Build history of the part. All positions in model axes, mm. Face numbers are marked on the shaded views. A direction names the side the tool comes from. Round coordinates to 2 decimals unless told otherwise and drop trailing zeros. Loops run counter-clockwise (first coordinate to the right, second up) from the corner with the lowest first, then second, coordinate; pieces in that order, holes last. Notation, with made-up numbers: (13.25, -37) - (43.25, -37) arc R22 ccw to (43.25, -20) - close; hole circle Ø3 at (-9.75, 81). An arc over 180 degrees is marked (long way). Use a Markdown table: item, result.
from build123d import *
from OCP.BRepFilletAPI import BRepFilletAPI_MakeChamfer

# Parameters (mm, degrees)
SKETCH1_R                    = 20
BOSS_EXTRUDE1_DEPTH          = 40
WRAP6_SECTION_W              = 2
WRAP6_SECTION_H              = 40
WRAP6_ANGLE                  = 68.754935416
CUT_EXTRUDE3_DEPTH           = 40
CUT_EXTRUDE4_DEPTH           = 40
SHELL1_START                 = -38.5
SHELL1_DEPTH                 = 37
BOSS_EXTRUDE6_DEPTH          = 1.7
CHAMFER3_SIZE2               = 5.104153638
CHAMFER3_SIZE                = 0.9
LPATTERN3_COUNT              = 7
LPATTERN3_PITCH              = 6.22
CHAMFER3_OF_LPATTERN3_SIZE   = 0.9
CHAMFER3_OF_LPATTERN3_SIZE_2 = 5.104153638
BOSS_EXTRUDE9_DEPTH          = 1.7
BOSS_EXTRUDE10_DEPTH         = 1.7
BOSS_EXTRUDE11_REACH         = 61.927
BOSS_EXTRUDE11_END_RADIUS    = 20
SKETCH26_W                   = 1.7
SKETCH26_H                   = 8.060132267
BOSS_EXTRUDE12_REACH         = 61.482
BOSS_EXTRUDE12_END_RADIUS    = 20
SKETCH31_W                   = 1.7
SKETCH31_H                   = 8.563925154
SKETCH35_R                   = 2.4
CUT_EXTRUDE5_DEPTH           = 46.6949855
SKETCH36_R                   = 3.1
CUT_EXTRUDE6_DEPTH           = 0.4
CUT_EXTRUDE7_START           = -0.4
SKETCH37_R                   = 3.1
CUT_EXTRUDE7_DEPTH           = 0.4
LPATTERN4_COUNT              = 2
LPATTERN4_PITCH              = 16
FILLET1_R                    = 4
BOSS_EXTRUDE13_DEPTH         = 0.4
LPATTERN5_COUNT              = 2
LPATTERN5_PITCH              = 40.1
SKETCH39_W                   = 40.5
SKETCH39_H                   = 1.5
BOSS_EXTRUDE14_DEPTH         = 1.5
SKETCH40_W                   = 40.5
SKETCH40_H                   = 1.5
BOSS_EXTRUDE15_DEPTH         = 2
BOSS_EXTRUDE15_TAPER         = 12


# Read off the part's stored shape, not the designer's step: Shell1
with BuildPart() as part:
    # Sketch1 → Boss-Extrude1 (new body)
    with BuildSketch(Plane(origin=(0, 0, 0), x_dir=(0, 0, -1), z_dir=(1, 0, 0))):
        Circle(SKETCH1_R)
    extrude(amount=-BOSS_EXTRUDE1_DEPTH)

    # Wrap6 section (on wrap section) → Wrap6 (revolve)
    with BuildSketch(Plane(origin=(0, 0, 0), x_dir=(0, 0.19866933079506122, 0.9800665778412416), z_dir=(0, 0.9800665778412416, -0.19866933079506122))):
        with Locations((21, -20)):
            Rectangle(WRAP6_SECTION_W, WRAP6_SECTION_H)
    revolve(axis=Axis((0, 0, 0), (1, 0, 0)), revolution_arc=WRAP6_ANGLE)

    # Sketch7 → Cut-Extrude3 (cut)
    with BuildSketch(Plane(origin=(0, 0, 0), x_dir=(0, 0, -1), z_dir=(1, 0, 0))):
        Polygon((-21.561464713, 4.370725277), (-10.806046117, -16.829419696), (-13.2224557, -32.299256077), (-33.361013034, 4.370725277), align=None)
    extrude(amount=-CUT_EXTRUDE3_DEPTH, mode=Mode.SUBTRACT)

    # Sketch8 → Cut-Extrude4 (cut)
    with BuildSketch(Plane(origin=(0, 0, 0), x_dir=(0, 0, -1), z_dir=(1, 0, 0))):
        with BuildLine():
            Line((-19.601331557, 3.973386616), (-17.669228411, 0))
            Line((-17.669228411, 0), (20, 0))
            ThreePointArc((20, 0), (1.996668333, 19.900083306), (-19.601331557, 3.973386616))
        make_face()
    extrude(amount=-CUT_EXTRUDE4_DEPTH, mode=Mode.SUBTRACT)

    # Shell1 outline → Shell1 (cut)
    with BuildSketch(Plane.YZ.offset(SHELL1_START)):
        with BuildLine():
            Line((0, 17.662079948), (-15.779750214, 9.656577198))
            ThreePointArc((-15.779750214, 9.656577198), (-16.138411913, -9.044427064), (0, -18.5))
            Line((0, -18.5), (0, 17.662079948))
        make_face()
    extrude(amount=SHELL1_DEPTH, mode=Mode.SUBTRACT)

    # Sketch17 → Boss-Extrude6 (add)
    with BuildSketch(Plane(origin=(0, -7.804938117, 15.384414667), x_dir=(1, 0, 0), z_dir=(0, -0.4524337453692514, 0.8917980186405168))):
        Polygon((-2.641259026, 11.553646958), (0, 11.553646958), (0, 13.652938378), (0, 17.652938378), (-2.641259026, 17.652938378), align=None)
    boss_extrude6 = extrude(amount=-BOSS_EXTRUDE6_DEPTH)

    # Chamfer3
    chamfer3_edges = [part.edges().sort_by_distance(p)[0] for p in [
        (-1.320629513, 8.707054719, 21.855143062),
    ]]
    chamfer3_side = [part.faces().sort_by_distance(p)[0] for p in [
        (-1.320629513, 8.698910912, 21.871195427),
    ]]
    chamfer(chamfer3_edges, length=CHAMFER3_SIZE - 0.0001, length2=CHAMFER3_SIZE2 - 0.0001, reference=chamfer3_side[0])  # a hair under: the kernel refuses the full size

    # LPattern3: Boss-Extrude6 ×7
    with Locations(*[(-i * LPATTERN3_PITCH, 0, 0) for i in range(1, LPATTERN3_COUNT)]):
        add(boss_extrude6)

    # Chamfer3 of LPattern3
    chamfer3_of_lpattern3_edges_1 = [part.edges().sort_by_distance(p)[0] for p in [
        (-7.540629513, 8.707054719, 21.855143062),
    ]]
    chamfer3_of_lpattern3_side_1 = [part.faces().sort_by_distance(p)[0] for p in [
        (-7.540629513, 8.698910912, 21.871195427),
    ]]
    chamfer3_of_lpattern3_edges_2 = [part.edges().sort_by_distance(p)[0] for p in [
        (-13.760629513, 8.707054719, 21.855143062),
    ]]
    chamfer3_of_lpattern3_side_2 = [part.faces().sort_by_distance(p)[0] for p in [
        (-13.760629513, 8.698910912, 21.871195427),
    ]]
    chamfer3_of_lpattern3_edges_3 = [part.edges().sort_by_distance(p)[0] for p in [
        (-19.980629513, 8.707054719, 21.855143062),
    ]]
    chamfer3_of_lpattern3_side_3 = [part.faces().sort_by_distance(p)[0] for p in [
        (-19.980629513, 8.698910912, 21.871195427),
    ]]
    chamfer3_of_lpattern3_edges_4 = [part.edges().sort_by_distance(p)[0] for p in [
        (-26.200629513, 8.707054719, 21.855143062),
    ]]
    chamfer3_of_lpattern3_side_4 = [part.faces().sort_by_distance(p)[0] for p in [
        (-26.200629513, 8.698910912, 21.871195427),
    ]]
    chamfer3_of_lpattern3_edges_5 = [part.edges().sort_by_distance(p)[0] for p in [
        (-32.420629513, 8.707054719, 21.855143062),
    ]]
    chamfer3_of_lpattern3_side_5 = [part.faces().sort_by_distance(p)[0] for p in [
        (-32.420629513, 8.698910912, 21.871195427),
    ]]
    chamfer3_of_lpattern3_edges_6 = [part.edges().sort_by_distance(p)[0] for p in [
        (-38.640629513, 8.707054719, 21.855143062),
    ]]
    chamfer3_of_lpattern3_side_6 = [part.faces().sort_by_distance(p)[0] for p in [
        (-38.640629513, 8.691002355, 21.846999255),
    ]]
    chamfer3_of_lpattern3 = BRepFilletAPI_MakeChamfer(part.part.solid().wrapped)
    for e in chamfer3_of_lpattern3_edges_1:
        chamfer3_of_lpattern3.Add(CHAMFER3_OF_LPATTERN3_SIZE - 0.0001, CHAMFER3_OF_LPATTERN3_SIZE_2 - 0.0001, e.wrapped, chamfer3_of_lpattern3_side_1[0].wrapped)
    for e in chamfer3_of_lpattern3_edges_2:
        chamfer3_of_lpattern3.Add(CHAMFER3_OF_LPATTERN3_SIZE - 0.0001, CHAMFER3_OF_LPATTERN3_SIZE_2 - 0.0001, e.wrapped, chamfer3_of_lpattern3_side_2[0].wrapped)
    for e in chamfer3_of_lpattern3_edges_3:
        chamfer3_of_lpattern3.Add(CHAMFER3_OF_LPATTERN3_SIZE - 0.0001, CHAMFER3_OF_LPATTERN3_SIZE_2 - 0.0001, e.wrapped, chamfer3_of_lpattern3_side_3[0].wrapped)
    for e in chamfer3_of_lpattern3_edges_4:
        chamfer3_of_lpattern3.Add(CHAMFER3_OF_LPATTERN3_SIZE - 0.0001, CHAMFER3_OF_LPATTERN3_SIZE_2 - 0.0001, e.wrapped, chamfer3_of_lpattern3_side_4[0].wrapped)
    for e in chamfer3_of_lpattern3_edges_5:
        chamfer3_of_lpattern3.Add(CHAMFER3_OF_LPATTERN3_SIZE - 0.0001, CHAMFER3_OF_LPATTERN3_SIZE_2 - 0.0001, e.wrapped, chamfer3_of_lpattern3_side_5[0].wrapped)
    for e in chamfer3_of_lpattern3_edges_6:
        chamfer3_of_lpattern3.Add(CHAMFER3_OF_LPATTERN3_SIZE_2 - 0.0001, CHAMFER3_OF_LPATTERN3_SIZE - 0.0001, e.wrapped, chamfer3_of_lpattern3_side_6[0].wrapped)
    add(Compound.cast(chamfer3_of_lpattern3.Shape()), mode=Mode.REPLACE)  # a hair under: the kernel refuses the full size



with BuildPart() as body_2:
    # Sketch18 → Boss-Extrude9 (new body)
    with BuildSketch(Plane(origin=(-12, 9.40212228, -3.028508389), x_dir=(0, -0.20791169081773309, -0.9781476007338114), z_dir=(1, 0, 0))):
        with BuildLine():
            Line((24.462887784, -6.44514078), (19.462887784, -6.44514078))
            Line((19.462887784, -6.44514078), (18.368989474, -14.430697657))
            Line((18.368989474, -14.430697657), (24.462887784, -13.44514078))
            ThreePointArc((24.462887784, -13.44514078), (27.962887784, -9.94514078), (24.462887784, -6.44514078))
        make_face()
    boss_extrude9 = extrude(amount=BOSS_EXTRUDE9_DEPTH)


with BuildPart() as body_3:
    # Sketch23 → Boss-Extrude10 (new body)
    with BuildSketch(Plane(origin=(-12, 6.645607303, -3.623209558), x_dir=(0, -0.3420201433256566, -0.9396926207859128), z_dir=(1, 0, 0))):
        with BuildLine():
            Line((23.775411733, -9.543929755), (18.775411733, -9.543929755))
            Line((18.775411733, -9.543929755), (16.378556498, -17.765602275))
            Line((16.378556498, -17.765602275), (23.775411733, -16.543929755))
            ThreePointArc((23.775411733, -16.543929755), (27.275411733, -13.043929755), (23.775411733, -9.543929755))
        make_face()
    boss_extrude10 = extrude(amount=BOSS_EXTRUDE10_DEPTH)


with BuildPart() as part_1:
    add(part.part)

    add(body_2.part)  # Boss-Extrude11 merges body 2
    # Boss-Extrude11: up to this cylinder (the profile starts outside it)
    boss_extrude11_end = Plane(origin=(-11.15, 0, 0), z_dir=(1, 0, 0)) * Cylinder(BOSS_EXTRUDE11_END_RADIUS, 164.854, mode=Mode.PRIVATE)
    # Sketch26 → Boss-Extrude11 (add, up to the surface)
    with BuildSketch(Plane(origin=(0, -6.71453374, -18.65024081), x_dir=(1, 0, 0), z_dir=(0, 0.3387394336586716, 0.9408802240905069)), mode=Mode.PRIVATE) as boss_extrude11_sk1:
        with Locations((-11.15, 2.098020073)):
            Rectangle(SKETCH26_W, SKETCH26_H)
    boss_extrude11_tool1 = extrude(boss_extrude11_sk1.sketch, amount=BOSS_EXTRUDE11_REACH, mode=Mode.PRIVATE) - boss_extrude11_end
    boss_extrude11 = boss_extrude11_tool1.solids().sort_by_distance((-11.15, -4.740548, -19.360923))[0]
    add(boss_extrude11)


    add(body_3.part)  # Boss-Extrude12 merges body 3
    # Boss-Extrude12: up to this cylinder (the profile starts outside it)
    boss_extrude12_end = Plane(origin=(-11.15, 0, 0), z_dir=(1, 0, 0)) * Cylinder(BOSS_EXTRUDE12_END_RADIUS, 163.964, mode=Mode.PRIVATE)
    # Sketch31 → Boss-Extrude12 (add, up to the surface)
    with BuildSketch(Plane(origin=(0, -11.64258856, -15.876784348), x_dir=(-1, 0, 0), z_dir=(0, -0.5913508934195582, -0.8064143605193862)), mode=Mode.PRIVATE) as boss_extrude12_sk1:
        with Locations((11.15, -0.687946115)):
            Rectangle(SKETCH31_W, SKETCH31_H)
    boss_extrude12_tool1 = extrude(boss_extrude12_sk1.sketch, amount=-BOSS_EXTRUDE12_REACH, mode=Mode.PRIVATE) - boss_extrude12_end
    boss_extrude12 = boss_extrude12_tool1.solids().sort_by_distance((-11.15, -12.197358, -15.469967))[0] + boss_extrude12_tool1.solids().sort_by_distance((-11.15, -12.197358, -15.469967))[1]
    add(boss_extrude12)

    # Sketch35 → Cut-Extrude5 (cut, through all)
    with BuildSketch(Plane(origin=(-10.3, 0, 0), x_dir=(0, 0, -1), z_dir=(1, 0, 0))):
        with Locations((24.889112346, -5.411813674)):
            Circle(SKETCH35_R)
        with Locations((21.503501796, -13.743346963)):
            Circle(SKETCH35_R)
    cut_extrude5 = extrude(amount=-CUT_EXTRUDE5_DEPTH, mode=Mode.SUBTRACT)

    # Sketch36 → Cut-Extrude6 (cut)
    with BuildSketch(Plane(origin=(-10.3, 0, 0), x_dir=(0, 0, -1), z_dir=(1, 0, 0))):
        with Locations((24.889112346, -5.411813674)):
            Circle(SKETCH36_R)
        with Locations((21.503501796, -13.743346963)):
            Circle(SKETCH36_R)
    cut_extrude6 = extrude(amount=-CUT_EXTRUDE6_DEPTH, mode=Mode.SUBTRACT)

    # Sketch37 → Cut-Extrude7 (cut)
    with BuildSketch(Plane.ZY.offset(12).offset(CUT_EXTRUDE7_START)):
        with Locations(Location((-24.889112346, -5.411813674, 0), (0, 0, 180))):
            Circle(SKETCH37_R)
        with Locations(Location((-21.503501796, -13.743346963, 0), (0, 0, 180))):
            Circle(SKETCH37_R)
    cut_extrude7 = extrude(amount=CUT_EXTRUDE7_DEPTH, mode=Mode.SUBTRACT)

    # LPattern4: Boss-Extrude9, Boss-Extrude10, Boss-Extrude11, Boss-Extrude12, Cut-Extrude5, Cut-Extrude6, Cut-Extrude7 ×2
    with Locations(*[(-i * LPATTERN4_PITCH, 0, 0) for i in range(1, LPATTERN4_COUNT)]):
        add(boss_extrude9)
        add(boss_extrude10)
        add(boss_extrude11)
        add(boss_extrude12)
        add(cut_extrude5, mode=Mode.SUBTRACT)
        add(cut_extrude6, mode=Mode.SUBTRACT)
        add(cut_extrude7, mode=Mode.SUBTRACT)

    # Fillet1
    fillet1_edges = [part_1.edges().sort_by_distance(p)[0] for p in [
        (-20, -16.829419696, 10.806046117),
    ]]
    fillet(fillet1_edges, radius=FILLET1_R)

    # Sketch38 → Boss-Extrude13 (add)
    with BuildSketch(Plane(origin=(0, 0, 0), x_dir=(0, 0, -1), z_dir=(1, 0, 0))):
        Polygon((-19.72457086, 0.75), (20, 0.75), (20, -0.75), (-16.900694448, -0.75), (-16.986407143, -4.647229987), align=None)
    boss_extrude13 = extrude(amount=BOSS_EXTRUDE13_DEPTH)

    # LPattern5: Boss-Extrude13 ×2
    with Locations(*[(-i * LPATTERN5_PITCH, 0, 0) for i in range(1, LPATTERN5_COUNT)]):
        add(boss_extrude13)

    # Sketch39 → Boss-Extrude14 (add)
    with BuildSketch(Plane(origin=(0, 0, -20), x_dir=(-1, 0, 0), z_dir=(0, 0, -1))):
        with Locations((19.85, 0)):
            Rectangle(SKETCH39_W, SKETCH39_H)
    extrude(amount=-BOSS_EXTRUDE14_DEPTH)

    # Sketch40 → Boss-Extrude15 (add)
    with BuildSketch(Plane(origin=(0, 0.75, 0), x_dir=(1, 0, 0), z_dir=(0, 1, 0))):
        with Locations((-19.85, 19.25)):
            Rectangle(SKETCH40_W, SKETCH40_H)
    extrude(amount=BOSS_EXTRUDE15_DEPTH, taper=BOSS_EXTRUDE15_TAPER)


solid = part_1.part
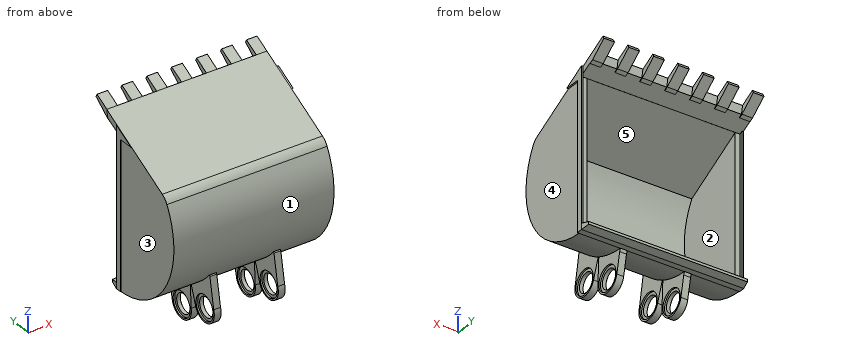
Q1. Which spindle directions (+Z, -Z, +X, -X, +Y, -Y) get a long thin tool onto all of the face, cutting with end or side? Do the marked faces 1, 2 and 3. Say none if no direction does.
Results found:
| item | result |
|---|---|
| face 1 | -Y |
| face 2 | +Y |
| face 3 | -Z, -X, -Y |
Q2. Cut at B-B, the plane z = -12. List the corners of the cut face in (x, y).
Results found:
| item | result |
|---|---|
| outline | (-40.1, -0.75) - (-40, -0.75) - (-40, -16) - (0, -16) - (0, -0.75) - (0.4, -0.75) - (0.4, 0.75) - (0, 0.75) - (0, 0) - (-1.5, 0) - (-1.5, -14.08) - (-38.5, -14.08) - (-38.5, 0) - (-39.7, 0) - (-39.7, 0.75) - (-40.1, 0.75) - close |
Q3. Cut at C-C, the plane z = 5. List the corners of the cut face in (x, y), plus the area to 3 significant figures.
Results found:
| item | result |
|---|---|
| outline | (-40.1, -0.75) - (-40, -0.75) - (-40, -19.36) - (0, -19.36) - (0, -0.75) - (0.4, -0.75) - (0.4, 0.75) - (0, 0.75) - (0, 0) - (-1.5, 0) - (-1.5, -17.81) - (-38.5, -17.81) - (-38.5, 0) - (-39.7, 0) - (-39.7, 0.75) - (-40.1, 0.75) - close |
| area | 117 mm2 |
Q4. Pull direction Z, two halves, no side cores. Call the marked faces 4 and 5: pulls with the +Z half, pulls with the -Z half, needs draft (parallel to the pull), parting line crosses it, or undercut.
Results found:
| item | result |
|---|---|
| face 4 | needs draft |
| face 5 | undercut |
Q5. Probe line 1 (X direction, y = -9.75, z = -13); line 2 (Z direction, x = -30, y = 1.5); line 3 (Z direction, x = -38, y = -5). List the from-to ranges inside material, lowest first.
Results found:
| item | result |
|---|---|
| line 1 | x = -40 to -38.5, -1.5 to 0 |
| line 2 | z = -19.84 to -18.66, 18.4 to 20.11 |
| line 3 | z = -19.36 to -17.81, 15.13 to 16.81 |
Q6. Cut at A-A, the plane y = 5.75. List the corners of the cut face in (x, z), plus the area to 3 significant figures.
Results found:
| item | result |
|---|---|
| outline | (-39.96, 20.74) - (-37.32, 20.74) - (-37.32, 22.26) - (-39.96, 22.26) - close; (-33.74, 20.74) - (-31.1, 20.74) - (-31.1, 22.26) - (-33.74, 22.26) - close; (-27.52, 20.74) - (-24.88, 20.74) - (-24.88, 22.26) - (-27.52, 22.26) - close; (-21.3, 20.74) - (-18.66, 20.74) - (-18.66, 22.26) - (-21.3, 22.26) - close; (-15.08, 20.74) - (-12.44, 20.74) - (-12.44, 22.26) - (-15.08, 22.26) - close; (-8.86, 20.74) - (-6.22, 20.74) - (-6.22, 22.26) - (-8.86, 22.26) - close; (-2.64, 20.74) - (0, 20.74) - (0, 22.26) - (-2.64, 22.26) - close |
| area | 28.1 mm2 |
Q7. Drop flat-ended pins along their axis: pin 1 (5.5 mm diameter, centred on y = -5.41, z = -24.89, fed in from -X); pin 2 (6 mm diameter, centred on x = -8.5, y = 2, fed in from +Z); pin 3 (1.9 mm diameter, centred on y = -12.5, z = -20, fed in from +X); pin 4 (3.5 mm diameter, centred on y = -5.41, z = -24.89, fed in from +X). Give the stop position or say it passes through.
Results found:
| item | result |
|---|---|
| pin 1 | stops at x = -27.6 |
| pin 2 | stops at z = 21.88 |
| pin 3 | stops at x = -10.7 |
| pin 4 | passes through |
